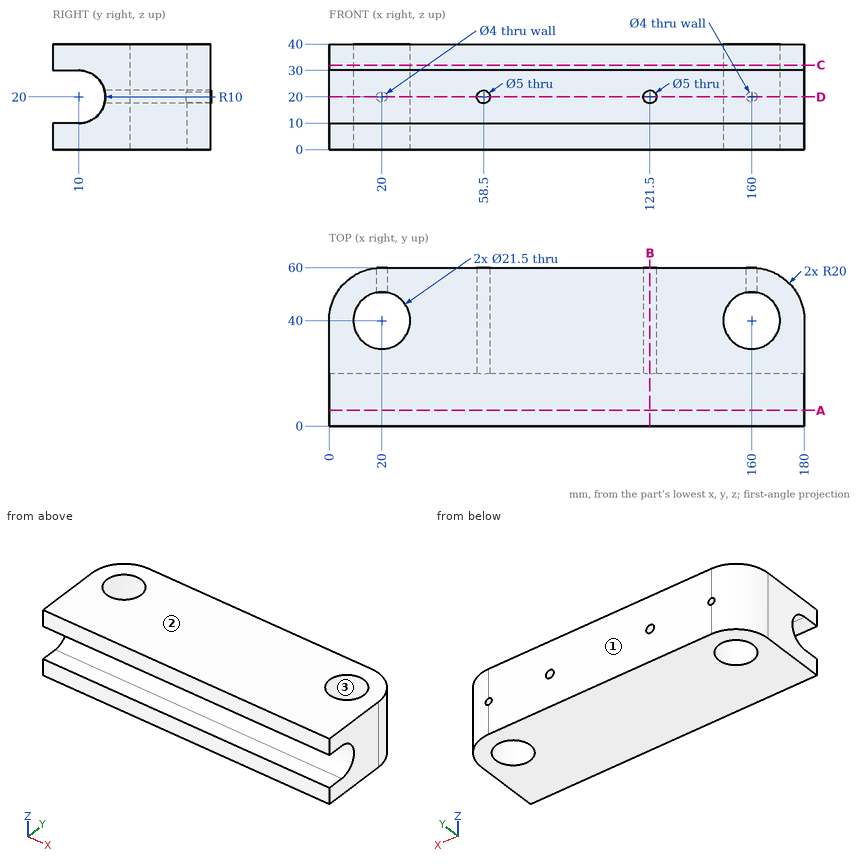
Geometry check sheet. Reference: drawing and pictorial views, mm from the part's lowest x, y, z. Give positions to 0.01 mm unless a question says otherwise; leave off trailing zeros. Order: outer loops, then holes, each group sorted by start corner. A loop starts at its lowest first (then second) coordinate and runs counter-clockwise, first axis right, second up. Notation, with made-up numbers: (6, 19.5) - (24, 19.5) arc R25 cw to (24, 33.5) - close; hole circle Ø2 at (25, 62). An arc over 180 degrees is marked (long way). Answer as CSV lines item,"result". Start each with the question number.
Item 1: Section check B-B, the plane x = 121.5. Record the boundary of the cut face in (y, z), plus the area to 3 significant figures.
Item 2: Material ranges on L1, parallel to Z at x = 121.5, y = 37; L2, parallel to X at y = 47, z = 4 (3 decimals); L3, parallel to X at y = 35.5, z = 4.5, recorded low to high.
Item 3: Section check C-C, the plane z = 32. Record the boundary of the cut face in (x, y).
Item 4: Mould release check, pull along Y, two halves, no side actions. Record for the marked faces 1, 2 and 3: released by +Y, released by -Y, zero draft, split by the parting line, or undercut.
Item 5: Section check D-D, the plane z = 20. Record the boundary of the cut face in (x, y), plus the area to 3 significant figures.
Item 6: Section check A-A, the plane y = 6. Record the boundary of the cut face in (x, z).
Item 7: Gauge pin test, flat ends, axial feed: pin 1 (4 mm diameter, centred on y = 52.5, z = 21, fed in from -X); pin 2 (3.5 mm diameter, centred on x = 20, z = 20, fed in from -Y); pin 3 (4 mm diameter, centred on x = 53, z = 13, fed in from -Y); pin 4 (8 mm diameter, centred on x = 50.5, z = 29, fed in from -Y). Record the tip position at first contact, or that the pin passes through.
Filled in:
1,outline,"(0, 0) - (60, 0) - (60, 17.5) - (19.68, 17.5) arc R10 cw to (10, 10) - (0, 10) - close; (0, 30) - (10, 30) arc R10 cw to (19.68, 22.5) - (60, 22.5) - (60, 40) - (0, 40) - close"
1,area,"1,840 mm^2"
2,L1,"0 to 17.5, 22.5 to 40"
2,L2,"1.265 to 11.841, 28.159 to 151.841, 168.159 to 178.735"
2,L3,"0 to 10.24, 29.76 to 150.24, 169.76 to 180"
3,outline,"(0, 0) - (180, 0) - (180, 40) arc R20 ccw to (160, 60) - (20, 60) arc R20 ccw to (0, 40) - close; hole circle Ø21.5 at (20, 40); hole circle Ø21.5 at (160, 40)"
4,face 1,"released by +Y"
4,face 2,"zero draft"
4,face 3,"undercut"
5,outline,"(0, 20) - (56, 20) - (56, 60) - (22, 60) - (22, 50.56) arc R10.75 cw (long way) to (18, 50.56) - (18, 59.9) arc R20 ccw to (0, 40) - close; (61, 20) - (119, 20) - (119, 60) - (61, 60) - close; (124, 20) - (180, 20) - (180, 40) arc R20 ccw to (162, 59.9) - (162, 50.56) arc R10.75 cw (long way) to (158, 50.56) - (158, 60) - (124, 60) - close"
5,area,"5,830 mm^2"
6,outline,"(0, 0) - (180, 0) - (180, 10) - (0, 10) - close; (0, 30) - (180, 30) - (180, 40) - (0, 40) - close"
7,pin 1,"x = 2.98"
7,pin 2,"y = 19.85"
7,pin 3,"y = 14.36"
7,pin 4,"y = 0"
